```python
from build123d import *

# Parameters (mm, degrees)
SKETCH1_W           = 130
SKETCH1_H           = 130
SKETCH1_R           = 31
SKETCH1_R_2         = 26
SKETCH1_R_3         = 24
BOSS_EXTRUDE2_DEPTH = 5
SKETCH2_R           = 31
SKETCH2_R_2         = 26
BOSS_EXTRUDE3_DEPTH = 5
SKETCH3_R           = 1.42
SKETCH3_R_2         = 3
CUT_EXTRUDE1_DEPTH  = 5
SKETCH4_R           = 3
CUT_EXTRUDE2_DEPTH  = 3


with BuildPart() as part:
    # Sketch1 → Boss-Extrude2 (new body)
    # profile 1 of 4: a face of its own
    with BuildSketch(Plane(origin=(0, 0, 0), x_dir=(1, 0, 0), z_dir=(0, 1, 0))):
        Rectangle(SKETCH1_W, SKETCH1_H)
        Circle(SKETCH1_R, mode=Mode.SUBTRACT)
    # profile 2 of 4: a face of its own
    with BuildSketch(Plane(origin=(0, 0, 0), x_dir=(1, 0, 0), z_dir=(0, 1, 0))):
        Circle(SKETCH1_R)
        Circle(SKETCH1_R_2, mode=Mode.SUBTRACT)
    # profile 3 of 4: a face of its own
    with BuildSketch(Plane(origin=(0, 0, 0), x_dir=(1, 0, 0), z_dir=(0, 1, 0))):
        Circle(SKETCH1_R_2)
        Circle(SKETCH1_R_3, mode=Mode.SUBTRACT)
    # profile 4 of 4: a face of its own
    with BuildSketch(Plane(origin=(0, 0, 0), x_dir=(1, 0, 0), z_dir=(0, 1, 0))):
        Circle(SKETCH1_R_3)
    extrude(amount=BOSS_EXTRUDE2_DEPTH)

    # Sketch2 → Boss-Extrude3 (add)
    with BuildSketch(Plane(origin=(0, 5, 0), x_dir=(1, 0, 0), z_dir=(0, 1, 0))):
        with Locations(Location((0, 0, 0), (0, 0, 270))):
            Circle(SKETCH2_R)
        with Locations(Location((0, 0, 0), (0, 0, 270))):
            Circle(SKETCH2_R_2, mode=Mode.SUBTRACT)
    extrude(amount=BOSS_EXTRUDE3_DEPTH)

    # Sketch3 → Cut-Extrude1 (cut)
    with BuildSketch(Plane(origin=(0, 5, 0), x_dir=(1, 0, 0), z_dir=(0, 1, 0))):
        with Locations(Location((0, 6.35, 0), (0, 0, 270))):
            Circle(SKETCH3_R)
        with Locations(Location((6.35, 0, 0), (0, 0, 270))):
            Circle(SKETCH3_R)
        with Locations(Location((0, -6.35, 0), (0, 0, 270))):
            Circle(SKETCH3_R)
        with Locations(Location((-6.35, 0, 0), (0, 0, 270))):
            Circle(SKETCH3_R)
        with Locations(Location((0, 0, 0), (0, 0, 270))):
            Circle(SKETCH3_R_2)
    extrude(amount=-CUT_EXTRUDE1_DEPTH, mode=Mode.SUBTRACT)

    # Sketch4 → Cut-Extrude2 (cut)
    with BuildSketch(Plane(origin=(0, 0, 0), x_dir=(-1, 0, 0), z_dir=(0, -1, 0))):
        with Locations(Location((-6.35, 0, 0), (0, 0, 90))):
            Circle(SKETCH4_R)
        with Locations(Location((0, 6.35, 0), (0, 0, 90))):
            Circle(SKETCH4_R)
        with Locations(Location((6.35, 0, 0), (0, 0, 90))):
            Circle(SKETCH4_R)
        with Locations(Location((0, -6.35, 0), (0, 0, 90))):
            Circle(SKETCH4_R)
    extrude(amount=-CUT_EXTRUDE2_DEPTH, mode=Mode.SUBTRACT)


solid = part.part
```
Build history of the part. All positions in model axes, mm. A direction names the side the tool comes from. Round coordinates to 2 decimals unless told otherwise and drop trailing zeros. Loops run counter-clockwise (first coordinate to the right, second up) from the corner with the lowest first, then second, coordinate; pieces in that order, holes last.
Item 1: Which spindle directions (+Z, -Z, +X, -X, +Y, -Y) get a long thin tool onto all of the face, cutting with end or side? Do faces 1 (the face through (-15.821, 7.465, -20.633)), 2 (the face through (0.132, 1.479, 9.347)), 3 (the face through (-21, 10, -16)). Say none if no direction does.
Item 2: Saw through at A-A (x = 22.5). List the corners of the cut face in (y, z).
Item 3: Saw through at B-B (z = -16). List the corners of the cut face in (x, y), then the cut area to 3 significant figures.
Item 4: Drill centre lines: line 1 along X through (y, z) = (2.1, 0); line 2 along X through (y, z) = (4.4, 0); line 3 along X through (y, z) = (8.9, 0). Where is each one in solid material? Low to high.
Item 5: Pin check, flat tips, straight feed: P1, Ø9.5, axis at x = -6.35, z = 0, coming from the +Y side; P2, Ø3.5, axis at x = 0, z = -6.35, coming from the -Y side. Stop position of each tip, or through.
Item 6: Saw through at C-C (z = -56). List the corners of the cut face in (x, y).
Item 7: Two-plate mould, pull along X, no slides. Class faces 4 (the face through (3.688, 1.479, -1.384)), 5 (the face through (-65, 2, 1)), 6 (the face through (30.736, 7.465, -4.036)): released by +X, released by -X, zero draft, split by the parting line, or undercut.
Worked answers:
1. face 1: +Y
1. face 2: -Y
1. face 3: +Z, -Z, +X, -X, +Y
2. outline: (0, -65) - (5, -65) - (5, -21.32) - (10, -21.32) - (10, -13.03) - (5, -13.03) - (5, 13.03) - (10, 13.03) - (10, 21.32) - (5, 21.32) - (5, 65) - (0, 65) - close
3. outline: (-65, 0) - (65, 0) - (65, 5) - (26.55, 5) - (26.55, 10) - (20.49, 10) - (20.49, 5) - (-20.49, 5) - (-20.49, 10) - (-26.55, 10) - (-26.55, 5) - (-65, 5) - close
3. area: 711 mm2
4. line 1: x = -65 to -9.35, -3.35 to -3, 3 to 3.35, 9.35 to 65
4. line 2: x = -65 to -7.77, -4.93 to -3, 3 to 4.93, 7.77 to 65
4. line 3: x = -31 to -26, 26 to 31
5. P1: stops at y = 5
5. P2: stops at y = 3
6. outline: (-65, 0) - (65, 0) - (65, 5) - (-65, 5) - close
7. face 4: undercut
7. face 5: released by -X
7. face 6: split by the parting line
